Read the model definition and answer for the solid it produces. Units are mm, in the model's axes. Face numbers are marked on the shaded views. Give positions to 0.01 mm unless a question says otherwise; leave off trailing zeros. Write each loop counter-clockwise with the first axis right and the second up, starting at its lowest first coordinate (ties: lowest second). Pieces come first, ordered by that corner, then holes. Notation, with made-up numbers: M -20,20 L 6,20 A26 cw 6,56 Z; hole C 56.5,29 d5. An arc over 180 degrees is marked long. Put each result on its own line as item: value.
from build123d import *

# Parameters (mm, degrees)
RESSALTO_EXTRUS_O1_DEPTH = 4
ESBO_O2_R                = 5.05
CORTE_EXTRUS_O1_DEPTH    = 4
M3_CLEARANCE_HOLE1_D     = 3.2


with BuildPart() as part:
    # Esboço1 → Ressalto-extrusão1 (new body)
    with BuildSketch(Plane.XY):
        with BuildLine():
            Line((95.202808527, -295.7159332), (112.09037792, -295.7159332))
            ThreePointArc((112.09037792, -295.7159332), (103.646593224, -313.7659332), (95.202808527, -295.7159332))
        make_face()
    extrude(amount=RESSALTO_EXTRUS_O1_DEPTH)

    # Esboço2 → Corte-extrusão1 (cut)
    with BuildSketch(Plane.XY.offset(4)):
        with Locations((103.646593224, -302.7659332)):
            Circle(ESBO_O2_R)
    extrude(amount=-CORTE_EXTRUS_O1_DEPTH, mode=Mode.SUBTRACT)

    # M3 Clearance Hole1 (through all)
    with Locations(Plane.XY.offset(4)):
        with Locations((95.681870132, -302.765933199), (111.611316315, -302.765933199), (103.646593224, -310.730656291), (103.646593224, -294.801210108)):
            Hole(M3_CLEARANCE_HOLE1_D / 2)


solid = part.part
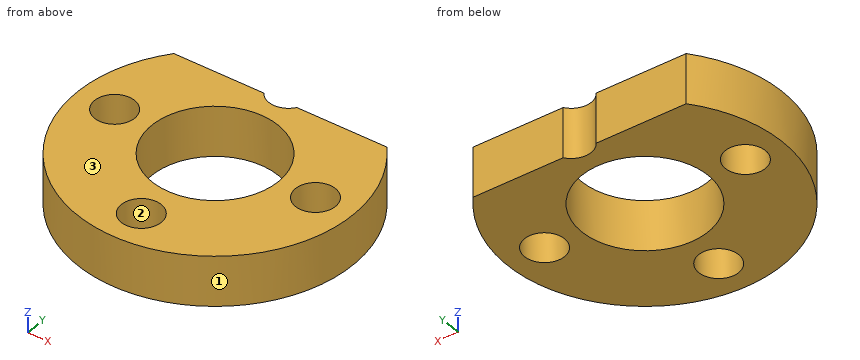
(1) Section D-D on x = 105.5 is taken. Determine the outline of the cut face in (y, z), and give its area (3 significant figures).
Result:
outline: M -313.61,0 L -307.46,0 L -307.46,4 L -313.61,4 Z; M -298.07,0 L -295.72,0 L -295.72,4 L -298.07,4 Z
area: 34.0 mm²
(2) Section B-B on x = 103.25 is taken. Determine the outline of the cut face in (y, z).
Result:
outline: M -313.76,0 L -312.28,0 L -312.28,4 L -313.76,4 Z; M -309.18,0 L -307.8,0 L -307.8,4 L -309.18,4 Z; M -297.73,0 L -296.35,0 L -296.35,4 L -297.73,4 Z
(3) For a pull along Y with two mould halves and no side action, classify the marked faces 1, 2 and 3 as +Y half, -Y half, draft (parallel to the pull), parting line (faces both ways), or undercut.
Result:
face 1: parting line
face 2: undercut
face 3: draft
(4) Section C-C on z = 3.15 is taken. Determine the outline of the cut face in (x, y), and give its area (3 significant figures).
Result:
outline: M 95.2,-295.72 A11 ccw long 112.09,-295.72 L 104.96,-295.72 A1.6 cw 102.33,-295.72 Z; hole C 95.68,-302.77 d3.2; hole C 103.65,-302.77 d10.1; hole C 103.65,-310.73 d3.2; hole C 111.61,-302.77 d3.2
area: 228 mm²
(5) Given pin 1 Ø6 at (x, y) = (103.65, -302.77) entering from +Z; pin 2 Ø1 at (x, z) = (95.5, 1.5) entering from -Y, each flat-ended and moving along its own axis, determine where each tip first touches the part or whether it passes through.
Result:
pin 1: passes through
pin 2: stops at y = -310.67
(6) Section A-A on y = -299.5 is taken. Determine the outline of the cut face in (x, z).
Result:
outline: M 93.14,0 L 99.79,0 L 99.79,4 L 93.14,4 Z; M 107.5,0 L 114.15,0 L 114.15,4 L 107.5,4 Z
(7) Straight lines are drawn through the part: line 1 along X through (y, z) = (-304, 2.45); line 2 along X through (y, z) = (-302, 2.9); line 3 along Y through (x, z) = (103.5, 3.7). For each, find the intervals that lie inside material, in ascending order. Write a range as from..to.
Result:
line 1: x = 92.72..94.66, 96.7..98.75, 108.54..110.59, 112.63..114.58
line 2: x = 92.67..94.28, 97.09..98.66, 108.64..110.21, 113.02..114.62
line 3: y = -313.76..-312.32, -309.14..-307.81, -297.72..-296.39
